from build123d import *

# Parameters (mm, degrees)
SKETCH1_R           = 12.5
BOSS_EXTRUDE1_DEPTH = 10
SKETCH2_R           = 7.5
CUT_EXTRUDE1_DEPTH  = 21.310096012
FILLET1_R           = 2


with BuildPart() as part:
    # Sketch1 → Boss-Extrude1 (new body)
    with BuildSketch(Plane(origin=(0, 0, 0), x_dir=(1, 0, 0), z_dir=(0, 1, 0))):
        with Locations(Location((0, 0, 0), (0, 0, 270))):
            Circle(SKETCH1_R)
    extrude(amount=BOSS_EXTRUDE1_DEPTH)

    # Sketch2 → Cut-Extrude1 (cut, through all)
    with BuildSketch(Plane(origin=(0, 10, 0), x_dir=(1, 0, 0), z_dir=(0, 1, 0))):
        with Locations(Location((0, 0, 0), (0, 0, 270))):
            Circle(SKETCH2_R)
    extrude(amount=-CUT_EXTRUDE1_DEPTH, mode=Mode.SUBTRACT)

    # Fillet1
    fillet1_edges = [part.edges().sort_by_distance(p)[0] for p in [
        (0, 0, -12.5),
        (0, 10, -12.5),
        (0, 0, -7.5),
        (0, 10, -7.5),
    ]]
    fillet(fillet1_edges, radius=FILLET1_R)


solid = part.part
Input: part model. Units: mm. Frame: model coordinates. Give positions to 0.01 mm unless a question says otherwise; leave off trailing zeros. Write each loop counter-clockwise with the first axis right and the second up, starting at its lowest first coordinate (ties: lowest second). Pieces come first, ordered by that corner, then holes.
Q1. Section B-B, the plane x = 0. Output: boundary loops of the cut face in (y, z).
Q2. First-contact query: P1, Ø1, axis at x = -2, y = 2, coming from the +Z side; P2, Ø5, axis at x = -3.5, z = 4.5, coming from the -Y side; P3, Ø1, axis at x = 2.5, y = 6, coming from the +Z side. Flat tips, straight axial feed; report the tip coordinate or a pass-through.
Q3. Section A-A, the plane z = 0. Output: boundary loops of the cut face in (x, y).
Q4. Section C-C, the plane y = 8.75. Output: boundary loops of the cut face in (x, z), plus the area to 3 significant figures.
Q5. Pull-direction query (X, two-part tool) for faces 1 (the face through (-9, 10, -5)), 2 (the face through (0.33, 5.042, -7.493)), 3 (the face through (3.755, 4.958, 11.923)); classes: pulls with the +X half, pulls with the -X half, needs draft (parallel to the pull), parting line crosses it, or undercut.
Q6. Material intervals for probe 1 along X at (y, z) = (5.3, 0); probe 2 along X at (y, z) = (2.5, -6); probe 3 along Z at (x, y) = (3, 6.5), sorted ascending.
Filled in:
1. outline: (0, -10.5) arc R2 ccw to (2, -12.5) - (8, -12.5) arc R2 ccw to (10, -10.5) - (10, -9.5) arc R2 ccw to (8, -7.5) - (2, -7.5) arc R2 ccw to (0, -9.5) - close; (0, 9.5) arc R2 ccw to (2, 7.5) - (8, 7.5) arc R2 ccw to (10, 9.5) - (10, 10.5) arc R2 ccw to (8, 12.5) - (2, 12.5) arc R2 ccw to (0, 10.5) - close
2. P1: stops at z = 12.41
2. P2: stops at y = 0.48
2. P3: stops at z = 12.34
3. outline: (-12.5, 2) arc R2 ccw to (-10.5, 0) - (-9.5, 0) arc R2 ccw to (-7.5, 2) - (-7.5, 8) arc R2 ccw to (-9.5, 10) - (-10.5, 10) arc R2 ccw to (-12.5, 8) - close; (7.5, 2) arc R2 ccw to (9.5, 0) - (10.5, 0) arc R2 ccw to (12.5, 2) - (12.5, 8) arc R2 ccw to (10.5, 10) - (9.5, 10) arc R2 ccw to (7.5, 8) - close
4. outline: circle Ø24.71 at (0, 0); hole circle Ø15.29 at (0, 0)
4. area: 296 mm2
5. face 1: needs draft
5. face 2: undercut
5. face 3: parting line crosses it
6. probe 1: x = -12.5 to -7.5, 7.5 to 12.5
6. probe 2: x = -10.97 to -4.5, 4.5 to 10.97
6. probe 3: z = -12.13 to -6.87, 6.87 to 12.13
